from build123d import *

# Parameters (mm, degrees)
SKETCH1_R           = 2.0025
BOSS_EXTRUDE1_DEPTH = 1.05
SKETCH3_R           = 1.5025
SKETCH3_W           = 5.005
SKETCH3_H           = 4.005
CUT_EXTRUDE8_DEPTH  = 0.85


with BuildPart() as part:
    # Sketch1 → Boss-Extrude1 (new body)
    with BuildSketch(Plane(origin=(0, 0, 0), x_dir=(1, 0, 0), z_dir=(0, 1, 0))):
        with BuildLine():
            Line((-69, 18.75), (-9, 18.75))
            Line((-9, 18.75), (-9, 17.65))
            Line((-9, 17.65), (-2.2, 17.65))
            Line((-2.2, 17.65), (-2.2, 18.75))
            Line((-2.2, 18.75), (4.8, 18.75))
            Line((4.8, 18.75), (4.8, 14.75))
            Line((4.8, 14.75), (9, 14.75))
            Line((9, 14.75), (9, 18.75))
            Line((9, 18.75), (69, 18.75))
            ThreePointArc((69, 18.75), (69.707106781, 18.457106781), (70, 17.75))
            Line((70, 17.75), (70, -17.75))
            ThreePointArc((70, -17.75), (69.707106781, -18.457106781), (69, -18.75))
            Line((69, -18.75), (-69, -18.75))
            ThreePointArc((-69, -18.75), (-69.707106781, -18.457106781), (-70, -17.75))
            Line((-70, -17.75), (-70, 17.75))
            ThreePointArc((-70, 17.75), (-69.707106781, 18.457106781), (-69, 18.75))
        make_face()
        with Locations((-65.35, -14.75)):
            Circle(SKETCH1_R, mode=Mode.SUBTRACT)
        with Locations((-60.25, -14.75)):
            Circle(SKETCH1_R, mode=Mode.SUBTRACT)
        with Locations((-55.15, -14.75)):
            Circle(SKETCH1_R, mode=Mode.SUBTRACT)
        with Locations((-50.05, -14.75)):
            Circle(SKETCH1_R, mode=Mode.SUBTRACT)
        with Locations((-44.95, -14.75)):
            Circle(SKETCH1_R, mode=Mode.SUBTRACT)
        with Locations((-39.85, -14.75)):
            Circle(SKETCH1_R, mode=Mode.SUBTRACT)
        with Locations((-34.75, -14.75)):
            Circle(SKETCH1_R, mode=Mode.SUBTRACT)
        with Locations((-29.65, -14.75)):
            Circle(SKETCH1_R, mode=Mode.SUBTRACT)
        with Locations((-24.55, -14.75)):
            Circle(SKETCH1_R, mode=Mode.SUBTRACT)
        with Locations((-19.45, -14.75)):
            Circle(SKETCH1_R, mode=Mode.SUBTRACT)
        with Locations((-14.35, -14.75)):
            Circle(SKETCH1_R, mode=Mode.SUBTRACT)
        with Locations((65.35, -14.75)):
            Circle(SKETCH1_R, mode=Mode.SUBTRACT)
        with Locations((60.25, -14.75)):
            Circle(SKETCH1_R, mode=Mode.SUBTRACT)
        with Locations((55.15, -14.75)):
            Circle(SKETCH1_R, mode=Mode.SUBTRACT)
        with Locations((50.05, -14.75)):
            Circle(SKETCH1_R, mode=Mode.SUBTRACT)
        with Locations((44.95, -14.75)):
            Circle(SKETCH1_R, mode=Mode.SUBTRACT)
        with Locations((39.85, -14.75)):
            Circle(SKETCH1_R, mode=Mode.SUBTRACT)
        with Locations((34.75, -14.75)):
            Circle(SKETCH1_R, mode=Mode.SUBTRACT)
        with Locations((29.65, -14.75)):
            Circle(SKETCH1_R, mode=Mode.SUBTRACT)
        with Locations((24.55, -14.75)):
            Circle(SKETCH1_R, mode=Mode.SUBTRACT)
        with Locations((19.45, -14.75)):
            Circle(SKETCH1_R, mode=Mode.SUBTRACT)
        with Locations((14.35, -14.75)):
            Circle(SKETCH1_R, mode=Mode.SUBTRACT)
    extrude(amount=-BOSS_EXTRUDE1_DEPTH)

    # Sketch3 → Cut-Extrude8 (cut)
    with BuildSketch(Plane.XZ.offset(1.05)):
        with Locations((62.23, -8.1425)):
            Circle(SKETCH3_R)
        with Locations((44.45, -8.1425)):
            Circle(SKETCH3_R)
        with Locations((26.67, -8.1425)):
            Circle(SKETCH3_R)
        with Locations((8.89, -8.1425)):
            Circle(SKETCH3_R)
        with Locations((-8.89, -8.1425)):
            Circle(SKETCH3_R)
        with Locations((-26.67, -8.1425)):
            Circle(SKETCH3_R)
        with Locations((-44.45, -8.1425)):
            Circle(SKETCH3_R)
        with Locations((-62.23, -8.1425)):
            Circle(SKETCH3_R)
        with Locations((62.2275, 0.7475)):
            Rectangle(SKETCH3_W, SKETCH3_H)
        with Locations((44.4475, 0.7475)):
            Rectangle(SKETCH3_W, SKETCH3_H)
        with Locations((26.6675, 0.7475)):
            Rectangle(SKETCH3_W, SKETCH3_H)
        with Locations((8.8875, 0.7475)):
            Rectangle(SKETCH3_W, SKETCH3_H)
        with Locations((-8.8925, 0.7475)):
            Rectangle(SKETCH3_W, SKETCH3_H)
        with Locations((-26.6725, 0.7475)):
            Rectangle(SKETCH3_W, SKETCH3_H)
        with Locations((-44.4525, 0.7475)):
            Rectangle(SKETCH3_W, SKETCH3_H)
        with Locations((-62.2325, 0.7475)):
            Rectangle(SKETCH3_W, SKETCH3_H)
    extrude(amount=-CUT_EXTRUDE8_DEPTH, mode=Mode.SUBTRACT)


solid = part.part
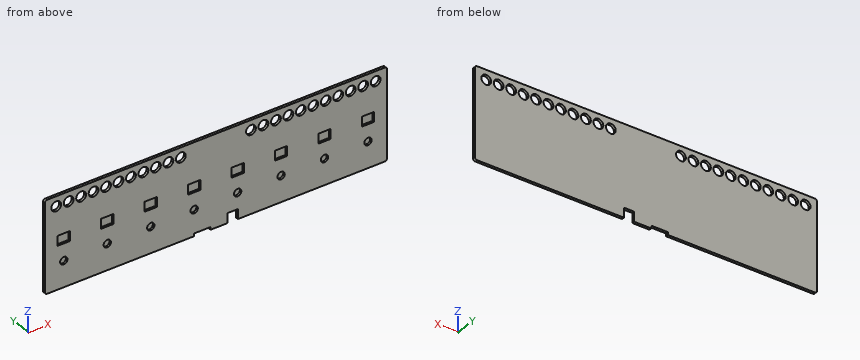
Design review of the part built by this model. Coordinates are the model's own, in mm. Give positions to 0.01 mm unless a question says otherwise; leave off trailing zeros. Order: outer loops, then holes, each group sorted by start corner. A loop starts at its lowest first (then second) coordinate and runs counter-clockwise, first axis right, second up.
1. For pin 1 Ø1.2 at (x, z) = (63, 1.5) entering from -Y, flat-tipped, find the tip position at first contact; note if it passes through.
Solution:
pin 1: stops at y = -0.2
2. Add section C-C, the plane x = -35.5. State the section outline as (y, z) points, then the cut area to 3 significant figures.
Solution:
outline: (-1.05, -18.75) - (0, -18.75) - (0, 12.89) - (-1.05, 12.89) - close; (-1.05, 16.61) - (0, 16.61) - (0, 18.75) - (-1.05, 18.75) - close
area: 35.5 mm2
3. To check wall thickness, follow L1, parallel to Z at x = -55, y = -0.7; L2, parallel to Z at x = 27, y = -0.3 (3 decimals). State the ranges of each line that lie inside material, in increasing order.
Solution:
L1: z = -18.75 to 12.75, 16.75 to 18.75
L2: z = -18.75 to -9.608, -6.677 to -1.255, 2.75 to 18.75
4. Add section A-A, the plane x = -14.35. State the section outline as (y, z) points.
Solution:
outline: (-1.05, -18.75) - (0, -18.75) - (0, 12.75) - (-1.05, 12.75) - close; (-1.05, 16.75) - (0, 16.75) - (0, 18.75) - (-1.05, 18.75) - close
5. Add section B-B, the plane y = -0.4. State how many separate pieces and enclosed holes the cut face has, then the cut area to 3 significant figures.
Solution:
separate pieces: 1
enclosed holes: 38
area: 4,730 mm2
